Verification items for this drawing (mm, ordinates from the low corner). A direction names the side the tool comes from. Round coordinates to 2 decimals unless told otherwise and drop trailing zeros. Loops run counter-clockwise (first coordinate to the right, second up) from the corner with the lowest first, then second, coordinate; pieces in that order, holes last. Notation, with made-up numbers: (75.25, 27.5) -> (80.25, 27.5) arc R14 ccw to (80.25, 54.5) -> close; hole circle Ø6 at (60.5, 80). An arc over 180 degrees is marked (long way). Use a Markdown table: item, result. Add a question column.
Q1. Set-up check for the marked faces 3, 4 and 5: record each of +Z, -Z, +X, -X, +Y, -Y from which the full face is reachable in a straight line by a thin tool's end or side.
Q2. Release check for a two-part mould opening along Z. For the marked faces 1 and 2 record: released by +Z, released by -Z, zero draft, split by the parting line, or undercut.
Q3. Sectioned sample at B-B, the plane x = 97. Enter the section's corners in (y, z).
Q4. Sectioned sample at C-C, the plane y = 15.25. Enter the section's corners in (x, z).
Q5. Sectioned sample at A-A, the plane z = 8. Enter the section's corners in (x, y).
Q6. Material ranges on L1, parallel to Z at x = 79, y = 22.25; L2, parallel to Y at x = 125.5, z = 24; L3, parallel to Y at x = 18.5, z = 3.25, recorded low to high.
Q7. Gauge pin test, flat ends, axial feed: P1, Ø6, axis at x = 8, z = 18, coming from the -Y side; P2, Ø12, axis at x = 132, y = 17.5, coming from the +Z side; P3, Ø7, axis at y = 16, z = 9, coming from the +X side; P4, Ø1.5, axis at x = 160, z = 13.5, coming from the +Y side. Record the tip position at first contact, or that the pin passes through.
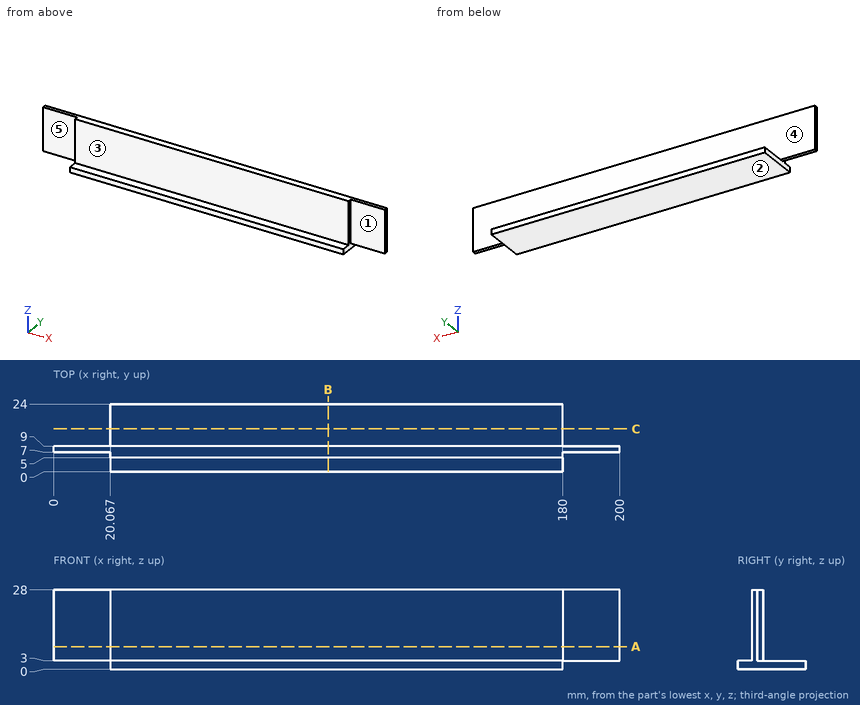
Values:
| question | item | result |
|---|---|---|
| 1 | face 3 | +Z, +X, -X, -Y |
| 1 | face 4 | +Z, +X, -X, +Y |
| 1 | face 5 | +Z, -Z, -X, -Y |
| 2 | face 1 | zero draft |
| 2 | face 2 | released by -Z |
| 3 | outline | (0, 0) -> (24, 0) -> (24, 3) -> (9, 3) -> (9, 28) -> (5, 28) -> (5, 3) -> (0, 3) -> close |
| 4 | outline | (20.07, 0) -> (180, 0) -> (180, 3) -> (20.07, 3) -> close |
| 5 | outline | (0, 7) -> (20.07, 7) -> (20.07, 5) -> (180, 5) -> (180, 7) -> (200, 7) -> (200, 9) -> (0, 9) -> close |
| 6 | L1 | 0 to 3 |
| 6 | L2 | 5 to 9 |
| 6 | L3 | 7 to 9 |
| 7 | P1 | y = 7 |
| 7 | P2 | z = 3 |
| 7 | P3 | through |
| 7 | P4 | y = 9 |
